Design review of the part built by this model. Coordinates are the model's own, in mm. A direction names the side the tool comes from. Round coordinates to 2 decimals unless told otherwise and drop trailing zeros. Loops run counter-clockwise (first coordinate to the right, second up) from the corner with the lowest first, then second, coordinate; pieces in that order, holes last. Notation, with made-up numbers: M -22.75,81.25 L 31.25,81.25 A20 ccw 31.25,93.25 Z; hole C -18,60.25 d8. An arc over 180 degrees is marked long. Use a Markdown table: item, result.
from build123d import *

# Parameters (mm, degrees)
BOSS_EXTRUDE1_DEPTH = 157.099
SKETCH2_R           = 3.2639
CUT_EXTRUDE1_DEPTH  = 12.7


with BuildPart() as part:
    # Sketch1 → Boss-Extrude1 (new body, symmetric)
    with BuildSketch(Plane(origin=(0, 0, 0), x_dir=(1, 0, 0), z_dir=(0, 1, 0))):
        Polygon((6.05685162, 4.132539387), (-0.550458281, 7.311657064), (-6.607309901, 3.179117677), (-6.05685162, -4.132539387), (0.550458281, -7.311657064), (6.607309901, -3.179117677), align=None)
    extrude(amount=BOSS_EXTRUDE1_DEPTH, both=True)

    # Sketch2 → Cut-Extrude1 (cut)
    with BuildSketch(Plane(origin=(0, 157.099, 0), x_dir=(1, 0, 0), z_dir=(0, 1, 0))):
        Circle(SKETCH2_R)
    cut_extrude1 = extrude(amount=-CUT_EXTRUDE1_DEPTH, mode=Mode.SUBTRACT)

    # Mirror1: Cut-Extrude1 across plane
    add(cut_extrude1.mirror(Plane.ZX), mode=Mode.SUBTRACT)


solid = part.part
1. Wall thickness on line 1 along Y through (x, z) = (1, 1); line 2 along Z through (x, y) = (0, -151.25); line 3 along X through (y, z) = (152.25, 0): over which ranges is each line inside the solid? List them lowest first. Write a range as from..to.
Check values:
| item | result |
|---|---|
| line 1 | y = -144.4..144.4 |
| line 2 | z = -7.05..-3.26, 3.26..7.05 |
| line 3 | x = -6.37..-3.26, 3.26..6.37 |
2. Take a section at B-B on z = 0. Give the boundary of the cut face in (x, y).
Check values:
| item | result |
|---|---|
| outline | M -6.37,-157.1 L -3.26,-157.1 L -3.26,-144.4 L 3.26,-144.4 L 3.26,-157.1 L 6.37,-157.1 L 6.37,157.1 L 3.26,157.1 L 3.26,144.4 L -3.26,144.4 L -3.26,157.1 L -6.37,157.1 Z |
3. The part is to be moulded in two halves that separate along Z. For faces 1 (the face through (0, -144.399, 0)), 2 (the face through (-3, 157.099, -2)), 3 (the face through (-3.5, 2.2, -5.3)), say which applies: pulls with the +Z half, pulls with the -Z half, needs draft (parallel to the pull), parting line crosses it, or undercut.
Check values:
| item | result |
|---|---|
| face 1 | undercut |
| face 2 | needs draft |
| face 3 | pulls with the -Z half |
4. Machinability: for faces 4 (the face through (-0.708, 150.838, 3.186)), 5 (the face through (-3, -157.099, -2)), 6 (the face through (-0.708, -150.838, 3.186)), which of the approach directions +Z, -Z, +X, -X, +Y, -Y give a long, thin tool a straight path to every point of the face, cutting with its end or side? Answer none if there is none.
Check values:
| item | result |
|---|---|
| face 4 | +Y |
| face 5 | +Z, -Z, +X, -X, -Y |
| face 6 | -Y |
5. Insertion check: pin 1 (5 mm diameter, centred on x = 0, z = 0, fed in from +Y); pin 2 (7 mm diameter, centred on x = -1, z = -1.5, fed in from -Y); pin 3 (5 mm diameter, centred on x = -3.5, y = -72, fed in from -Z); pin 4 (3 mm diameter, centred on y = 31.5, z = -4.5, fed in from +X). Each pin has a flat end and moves straight along its axis. Give the tip position at first contact, or say it passes through.
Check values:
| item | result |
|---|---|
| pin 1 | stops at y = 144.4 |
| pin 2 | stops at y = -157.1 |
| pin 3 | stops at z = -7 |
| pin 4 | stops at x = 6.14 |
6. Take a section at A-A on y = 16. Give the boundary of the cut face in (x, z), and give its area (3 significant figures).
Check values:
| item | result |
|---|---|
| outline | M -6.61,-3.18 L -0.55,-7.31 L 6.06,-4.13 L 6.61,3.18 L 0.55,7.31 L -6.06,4.13 Z |
| area | 140 mm² |
